Answer from the drawing. Dimensions are ordinates in mm from the lowest x, y and z of the part. A direction names the side the tool comes from. Round coordinates to 2 decimals unless told otherwise and drop trailing zeros. Loops run counter-clockwise (first coordinate to the right, second up) from the corner with the lowest first, then second, coordinate; pieces in that order, holes last. Notation, with made-up numbers: (-1.75, 36) - (49.25, 36) arc R24 cw to (49.25, 54) - close; hole circle Ø5 at (-31.5, 13.5). An arc over 180 degrees is marked (long way). Answer as CSV lines item,"result". Start each with the question number.
Q1. Section D-D on x = 13 is taken. Write down the section's boundary in (y, z), then the cut area to 3 significant figures.
Q2. Section B-B on z = 248 is taken. Write down the section's boundary in (x, y).
Q3. Straight lines are drawn through the part: L1, parallel to Y at x = 9.5, z = 460.5; L2, parallel to Y at x = 29, z = 327.5. For each, find the intervals that lie inside material, in ascending order. Write a range as [from, to].
Q4. Section C-C on y = 110 is taken. Write down the section's boundary in (x, z), then the cut area to 3 significant figures.
Q5. This flat-tipped pin is pushed along its axis until it touches: pin 1 Ø2 at (x, z) = (60, 74.5) entering from -Y. Where does it stop, or does it pass through?
Q6. For the marked faces 1 and 2, determine the directions among +Z, -Z, +X, -X, +Y, -Y from which every point of the face is accessible in a straight line to the end or side of a thin tool.
Q7. Section A-A on x = 60 is taken. Write down the section's boundary in (y, z), then the cut area to 3 significant figures.
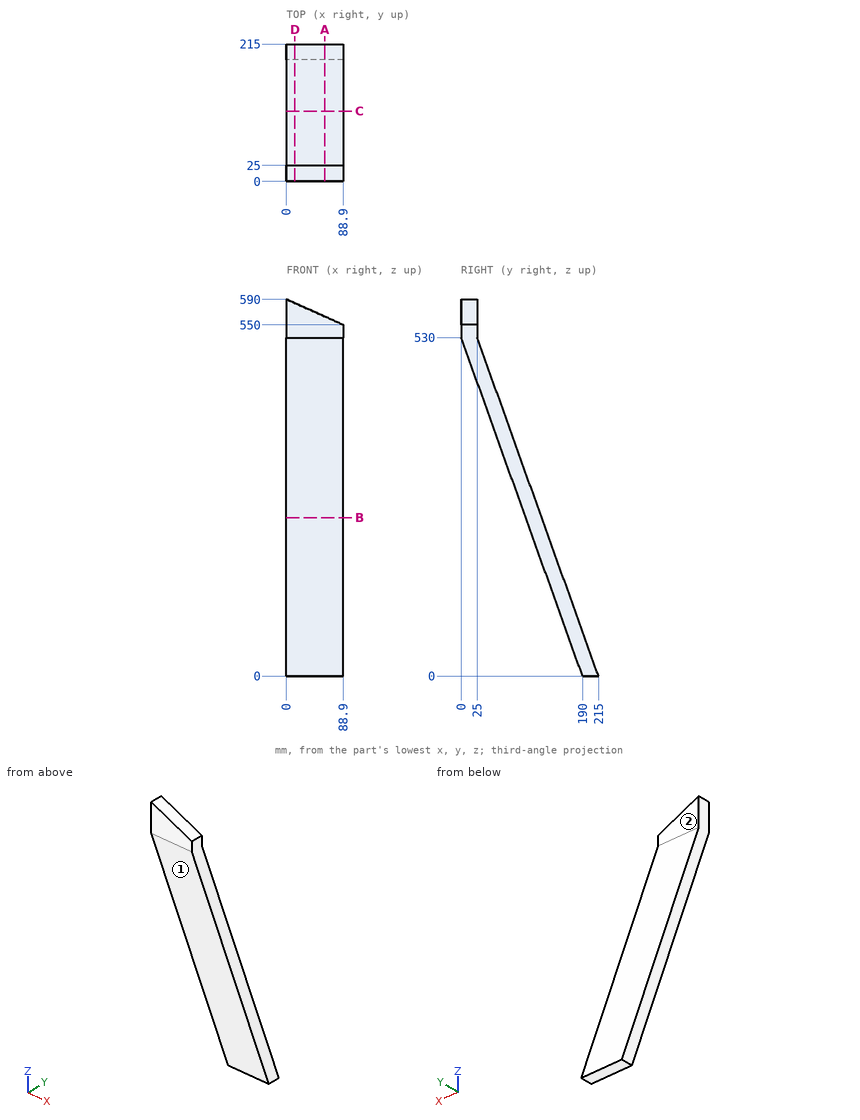
Findings:
1,outline,"(0, 530) - (190, 0) - (215, 0) - (25, 530) - (25, 584.15) - (0, 584.15) - close"
1,area,"14,600 mm^2"
2,outline,"(0, 101.09) - (88.9, 101.09) - (88.9, 126.09) - (0, 126.09) - close"
3,L1,"y = [24.92, 49.92]"
3,L2,"y = [72.59, 97.59]"
4,outline,"(0, 223.16) - (88.9, 223.16) - (88.9, 292.89) - (0, 292.89) - close"
4,area,"6,200 mm^2"
5,pin 1,"stops at y = 162.93"
6,face 1,"-Z, +X, -X, -Y"
6,face 2,"+Z, +X, -X, +Y"
7,outline,"(0, 530) - (190, 0) - (215, 0) - (25, 530) - (25, 563) - (0, 563) - close"
7,area,"14,100 mm^2"
